from build123d import *

# Parameters (mm, degrees)
SKETCH1_W           = 10
SKETCH1_H           = 5
BOSS_EXTRUDE1_DEPTH = 5
SKETCH2_W           = 5
SKETCH2_H           = 10
SKETCH2_H_2         = 15
BOSS_EXTRUDE2_DEPTH = 5
SKETCH3_R           = 2.5
SKETCH3_R_2         = 1.5
CUT_EXTRUDE1_DEPTH  = 298.573520327
CUT_EXTRUDE2_DEPTH  = 298.573520327
FILLET1_R           = 4


with BuildPart() as part:
    # Sketch1 → Boss-Extrude1 (new body)
    with BuildSketch(Plane(origin=(0, 0, 0), x_dir=(0, 0, -1), z_dir=(1, 0, 0))):
        Polygon((-50, 50), (-50, 55), (-20, 270), (0, 270), (0, 55), (0, 50), (0, 0), (-120, 0), (-120, 50), align=None)
        with Locations((-15, 52.5)):
            Rectangle(SKETCH1_W, SKETCH1_H, mode=Mode.SUBTRACT)
    extrude(amount=BOSS_EXTRUDE1_DEPTH)

    # Sketch2 → Boss-Extrude2 (add)
    with BuildSketch(Plane(origin=(5, 0, 0), x_dir=(0, 0, -1), z_dir=(1, 0, 0))):
        with Locations((-122.5, 10)):
            Rectangle(SKETCH2_W, SKETCH2_H)
        with Locations((-122.5, 40)):
            Rectangle(SKETCH2_W, SKETCH2_H)
        with Locations((2.5, 257.5)):
            Rectangle(SKETCH2_W, SKETCH2_H_2)
        with Locations((2.5, 77.5)):
            Rectangle(SKETCH2_W, SKETCH2_H_2)
        with Locations((2.5, 40)):
            Rectangle(SKETCH2_W, SKETCH2_H)
        with Locations((2.5, 10)):
            Rectangle(SKETCH2_W, SKETCH2_H)
        with Locations((2.5, 167.5)):
            Rectangle(SKETCH2_W, SKETCH2_H_2)
    extrude(amount=-BOSS_EXTRUDE2_DEPTH)

    # Sketch3 → Cut-Extrude1 (cut, through all)
    with BuildSketch(Plane(origin=(5, 0, 0), x_dir=(0, 0, -1), z_dir=(1, 0, 0))):
        with Locations((-41.4, 26.3)):
            Circle(SKETCH3_R)
        with Locations((-8, 212.5)):
            Circle(SKETCH3_R_2)
        with Locations((-8, 152.5)):
            Circle(SKETCH3_R_2)
        Polygon((0, 26.5), (-5, 26.5), (-5, 27.75), (-8, 27.75), (-8, 26.5), (-10, 26.5), (-10, 23.5), (-8, 23.5), (-8, 22.25), (-5, 22.25), (-5, 23.5), (0, 23.5), align=None)
        Polygon((0, 104), (-5, 104), (-5, 105.25), (-8, 105.25), (-8, 104), (-10, 104), (-10, 101), (-8, 101), (-8, 99.75), (-5, 99.75), (-5, 101), (0, 101), align=None)
        Polygon((0, 234), (-5, 234), (-5, 235.25), (-8, 235.25), (-8, 234), (-10, 234), (-10, 231), (-8, 231), (-8, 229.75), (-5, 229.75), (-5, 231), (0, 231), align=None)
        Polygon((-120, 23.5), (-120, 26.5), (-115, 26.5), (-115, 27.75), (-112, 27.75), (-112, 26.5), (-110, 26.5), (-110, 23.5), (-112, 23.5), (-112, 22.25), (-115, 22.25), (-115, 23.5), align=None)
        with BuildLine():
            Line((-3, 137.5), (-3, 122.5))
            ThreePointArc((-3, 122.5), (-8, 117.5), (-13, 122.5))
            Line((-13, 122.5), (-13, 137.5))
            ThreePointArc((-13, 137.5), (-8, 142.5), (-3, 137.5))
        make_face()
    extrude(amount=-CUT_EXTRUDE1_DEPTH, mode=Mode.SUBTRACT)

    # Sketch4 → Cut-Extrude2 (cut, through all)
    with BuildSketch(Plane(origin=(5, 0, 0), x_dir=(0, 0, -1), z_dir=(1, 0, 0))):
        with BuildLine():
            Line((-97, 38.5), (-97, 11.5))
            ThreePointArc((-97, 11.5), (-98.5, 10), (-100, 11.5))
            Line((-100, 11.5), (-100, 38.5))
            ThreePointArc((-100, 38.5), (-98.5, 40), (-97, 38.5))
        make_face()
        with BuildLine():
            Line((-91, 38.5), (-91, 11.5))
            ThreePointArc((-91, 11.5), (-92.5, 10), (-94, 11.5))
            Line((-94, 11.5), (-94, 38.5))
            ThreePointArc((-94, 38.5), (-92.5, 40), (-91, 38.5))
        make_face()
        with BuildLine():
            Line((-85, 38.5), (-85, 11.5))
            ThreePointArc((-85, 11.5), (-86.5, 10), (-88, 11.5))
            Line((-88, 11.5), (-88, 38.5))
            ThreePointArc((-88, 38.5), (-86.5, 40), (-85, 38.5))
        make_face()
        with BuildLine():
            Line((-79, 38.5), (-79, 11.5))
            ThreePointArc((-79, 11.5), (-80.5, 10), (-82, 11.5))
            Line((-82, 11.5), (-82, 38.5))
            ThreePointArc((-82, 38.5), (-80.5, 40), (-79, 38.5))
        make_face()
        with BuildLine():
            Line((-73, 38.5), (-73, 11.5))
            ThreePointArc((-73, 11.5), (-74.5, 10), (-76, 11.5))
            Line((-76, 11.5), (-76, 38.5))
            ThreePointArc((-76, 38.5), (-74.5, 40), (-73, 38.5))
        make_face()
        with BuildLine():
            Line((-67, 38.5), (-67, 11.5))
            ThreePointArc((-67, 11.5), (-68.5, 10), (-70, 11.5))
            Line((-70, 11.5), (-70, 38.5))
            ThreePointArc((-70, 38.5), (-68.5, 40), (-67, 38.5))
        make_face()
        with BuildLine():
            Line((-61, 38.5), (-61, 11.5))
            ThreePointArc((-61, 11.5), (-62.5, 10), (-64, 11.5))
            Line((-64, 11.5), (-64, 38.5))
            ThreePointArc((-64, 38.5), (-62.5, 40), (-61, 38.5))
        make_face()
        with BuildLine():
            Line((-55, 38.5), (-55, 11.5))
            ThreePointArc((-55, 11.5), (-56.5, 10), (-58, 11.5))
            Line((-58, 11.5), (-58, 38.5))
            ThreePointArc((-58, 38.5), (-56.5, 40), (-55, 38.5))
        make_face()
    extrude(amount=-CUT_EXTRUDE2_DEPTH, mode=Mode.SUBTRACT)

    # Fillet1
    fillet1_edges = [part.edges().sort_by_distance(p)[0] for p in [
        (2.5, 270, 20),
    ]]
    fillet(fillet1_edges, radius=FILLET1_R)


solid = part.part
For this review, take the finished solid that the model builds, in its own axes (mm). A direction names the side the tool comes from. Round coordinates to 2 decimals unless told otherwise and drop trailing zeros. Loops run counter-clockwise (first coordinate to the right, second up) from the corner with the lowest first, then second, coordinate; pieces in that order, holes last. Notation, with made-up numbers: (43.25, 20) - (100.25, 20) arc R25 ccw to (100.25, 54) - close; hole circle Ø11 at (-30.5, 87). An arc over 180 degrees is marked (long way). One line per item, written item: value. Start each with the question number.
Item 1: Take a section at C-C (y = 91.5). Give the boundary of the cut face in (x, z).
Item 2: For faces 1 (the flat face through (3, 160, -2)), 2 (the flat face through (3, 130, 3)), 3 (the flat face through (3, 257, -5)), 4 (the flat face through (2, 19, 120)), list the 3-axis set-ups (+Z, -Z, +X, -X, +Y, -Y) from which the entire face can be reached by the end or side of a thin tool; tool diameter is ignored.
Item 3: The part is to be moulded in two halves that separate along Y. For faces 5 (the flat face through (3, 25, 85)), 6 (the flat face through (2, 47, 120)), say which applies: +Y half, -Y half, draft (parallel to the pull), parting line (faces both ways), or undercut.
Item 4: For L1, parallel to Y at x = 1.3, z = 1.5; L2, parallel to Y at x = 1, z = 56.5; L3, parallel to Z at x = 3.25, y = 51, list the stretches that pass through material, from the lowest coordinate up.
Item 5: Take a section at A-A (z = 41.4). Give the boundary of the cut face in (x, y), plus the area to 3 significant figures.
Item 6: Clearance check with flat-ended pins moving along their axes: pin 1 Ø0.6 at (x, y) = (2.5, 235) entering from -Z; pin 2 Ø1.5 at (x, z) = (2, -2.5) entering from -Y; pin 3 Ø1.4 at (x, y) = (1.5, 27) entering from +Z. State where each tip first meets the part, or that it passes through.
Item 7: Take a section at B-B (x = 2.4). State how many separate pieces and enclosed holes the cut face has, plus the area to 3 significant figures.
Answer below:
1. outline: (0, 0) - (5, 0) - (5, 44.91) - (0, 44.91) - close
2. face 1: -Z, +X, -X
2. face 2: +X, -X
2. face 3: -Z, +X, -X, +Y, -Y
2. face 4: +Z, +X, -X
3. face 5: undercut
3. face 6: draft
4. L1: y = 0 to 23.5, 26.5 to 101, 104 to 231, 234 to 270
4. L2: y = 0 to 10, 40 to 50
4. L3: z = 0 to 10, 20 to 50
5. outline: (0, 0) - (5, 0) - (5, 23.8) - (0, 23.8) - close; (0, 28.8) - (5, 28.8) - (5, 116.63) - (0, 116.63) - close
5. area: 558 mm2
6. pin 1: stops at z = 0
6. pin 2: stops at y = 5
6. pin 3: stops at z = 120
7. separate pieces: 1
7. enclosed holes: 13
7. area: 13,000 mm2
